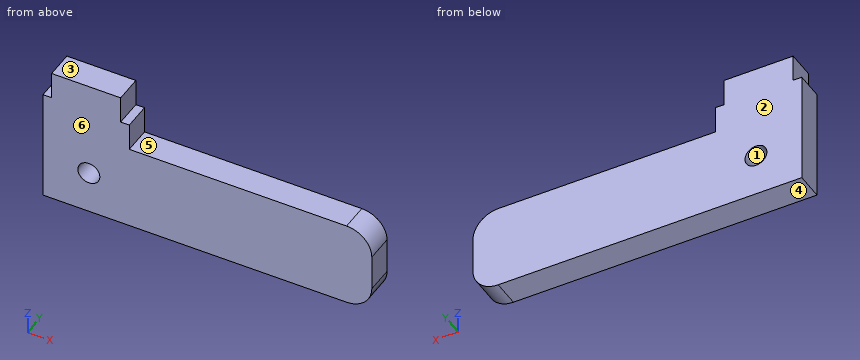
```python
from build123d import *

# Parameters (mm, degrees)
SKETCH1_R           = 1.27
BOSS_EXTRUDE1_DEPTH = 3.175
FILLET1_R           = 2.921
SKETCH2_W           = 1
SKETCH2_H           = 3.175
CUT_EXTRUDE1_DEPTH  = 42.583369873


with BuildPart() as part:
    # Sketch1 → Boss-Extrude1 (new body)
    with BuildSketch(Plane(origin=(0, 0, 0), x_dir=(1, 0, 0), z_dir=(0, 1, 0))):
        Polygon((0, 0), (0, 16.355), (38.1, 16.355), (38.1, 6.355), (10, 6.355), (10, 0), align=None)
        with Locations(Location((5.313, 11.35, 0), (0, 0, 270))):
            Circle(SKETCH1_R, mode=Mode.SUBTRACT)
    extrude(amount=BOSS_EXTRUDE1_DEPTH)

    # Fillet1
    fillet1_edges = [part.edges().sort_by_distance(p)[0] for p in [
        (38.1, 1.5875, -16.355),
        (38.1, 1.5875, -6.355),
    ]]
    fillet(fillet1_edges, radius=FILLET1_R)

    # Sketch2 → Cut-Extrude1 (cut, through all)
    with BuildSketch(Plane(origin=(0, 3.175, 0), x_dir=(1, 0, 0), z_dir=(0, 1, 0))):
        with Locations((9.5, 1.5875)):
            Rectangle(SKETCH2_W, SKETCH2_H)
        with Locations((0.5, 1.5875)):
            Rectangle(SKETCH2_W, SKETCH2_H)
    extrude(amount=-CUT_EXTRUDE1_DEPTH, mode=Mode.SUBTRACT)


solid = part.part
```
Could you check a few things on this model? Use its own coordinates, in mm. Face numbers are marked on the shaded views. A direction names the side the tool comes from. Give positions to 0.01 mm unless a question says otherwise; leave off trailing zeros. Loops run counter-clockwise (first coordinate to the right, second up) from the corner with the lowest first, then second, coordinate; pieces in that order, holes last. Notation, with made-up numbers: (46, 17) - (82, 17) arc R23 ccw to (82, 25) - close; hole circle Ø5 at (73.25, -7). An arc over 180 degrees is marked (long way). Answer in a Markdown table with one row per item. Add a question column.
Q1. We'd pull the mould along Z, two halves only. Please class the marked faces 1, 2, 3 and 4: +Z half, -Z half, draft (parallel to the pull), parting line (faces both ways), or undercut.
Q2. Please list where these lines run through material, in increasing order: L1, parallel to X at y = 0.7, z = -11.35; L2, parallel to Z at x = 13, y = 1.7 (3 decimals); L3, parallel to X at y = 1.05, z = -6.25. Write a range as from..to.
Q3. For pin 1 (1 mm diameter, centred on y = 2, z = -1, fed in from -X); pin 2 (1 mm diameter, centred on y = 2, z = -4.5, fed in from +X), each with a flat end and sliding along its axis, tell me the tip position at first contact or that it passes through.
Q4. If we section it at A-A (z = -11.35): List the corners of the cut face in (x, y) for me (3 decimals), plus the area to 3 significant figures.
Q5. If we section it at D-D (x = 30): List the corners of the cut face in (y, z) for me (3 decimals).
Q6. If we section it at B-B (x = 6): List the corners of the cut face in (y, z) for me (3 decimals).
Q7. Which directions (+Z, -Z, +X, -X, +Y, -Y) give clear straight access to the entire face, cutting with the end or side of a thin tool? Please do the marked faces 5 and 6.
Q8. If we section it at C-C (y = 1.55): List the corners of the cut face in (x, z) for me (3 decimals), plus the area to 3 significant figures.
The answers:
| question | item | result |
|---|---|---|
| 1 | face 1 | undercut |
| 1 | face 2 | draft |
| 1 | face 3 | +Z half |
| 1 | face 4 | -Z half |
| 2 | L1 | x = 0..4.04, 6.58..38.1 |
| 2 | L2 | z = -16.355..-6.355 |
| 2 | L3 | x = 0..10 |
| 3 | pin 1 | stops at x = 1 |
| 3 | pin 2 | stops at x = 10 |
| 4 | outline | (0, 0) - (4.043, 0) - (4.043, 3.175) - (0, 3.175) - close; (6.583, 0) - (38.1, 0) - (38.1, 3.175) - (6.583, 3.175) - close |
| 4 | area | 113 mm^2 |
| 5 | outline | (0, -16.355) - (3.175, -16.355) - (3.175, -6.355) - (0, -6.355) - close |
| 6 | outline | (0, -16.355) - (3.175, -16.355) - (3.175, -12.418) - (0, -12.418) - close; (0, -10.282) - (3.175, -10.282) - (3.175, 0) - (0, 0) - close |
| 7 | face 5 | +Z, +X, +Y, -Y |
| 7 | face 6 | +Z, -Z, +X, -X, -Y |
| 8 | outline | (0, -16.355) - (35.179, -16.355) arc R2.921 ccw to (38.1, -13.434) - (38.1, -9.276) arc R2.921 ccw to (35.179, -6.355) - (10, -6.355) - (10, -3.175) - (9, -3.175) - (9, 0) - (1, 0) - (1, -3.175) - (0, -3.175) - close; hole circle Ø2.54 at (5.313, -11.35) |
| 8 | area | 429 mm^2 |
